Verification items for the finished model (mm, model axes). Face numbers are marked on the shaded views. A direction names the side the tool comes from. Give positions to 0.01 mm unless a question says otherwise; leave off trailing zeros. Order: outer loops, then holes, each group sorted by start corner. A loop starts at its lowest first (then second) coordinate and runs counter-clockwise, first axis right, second up.
from build123d import *

# Parameters (mm, degrees)
F1_DEPTH = 15
F2_R     = 2
F3_DEPTH = 5
F4_R     = 4
F5_R     = 2.1


with BuildPart() as f1:
    # F0 (on Top) → F1 (new body)
    with BuildSketch(Plane.XY):
        with BuildLine():
            ThreePointArc((3, -2.645751), (-3.741657, 1.414214), (4, 0))
            Line((4, 0), (4, -20.91608))
            Line((4, -20.91608), (6, -20.91608))
            Line((6, -20.91608), (6, 0))
            ThreePointArc((6, 0), (-4.582576, 3.872983), (1, -5.91608))
            Line((1, -5.91608), (1, -20.91608))
            Line((1, -20.91608), (3, -20.91608))
            Line((3, -20.91608), (3, -2.645751))
        make_face()
    extrude(amount=F1_DEPTH)

    # F2 (on face) → F3 (cut, through all)
    with BuildSketch(Plane(origin=(1, 0, 0), x_dir=(0, -1, 0), z_dir=(-1, 0, 0))):
        with Locations((13.41608, 7.5)):
            Circle(F2_R)
    extrude(amount=-F3_DEPTH, mode=Mode.SUBTRACT)

    # F4 (on face) → F6 section 0
    with BuildSketch(Plane(origin=(1, 0, 0), x_dir=(0, -1, 0), z_dir=(-1, 0, 0))):
        with Locations((13.41608, 7.5)):
            Circle(F4_R)
    # F5 (on face) → F6 section 1
    with BuildSketch(Plane.YZ.offset(3)):
        with Locations((-13.41608, 7.5)):
            Circle(F5_R)
    loft(mode=Mode.SUBTRACT)


solid = f1.part
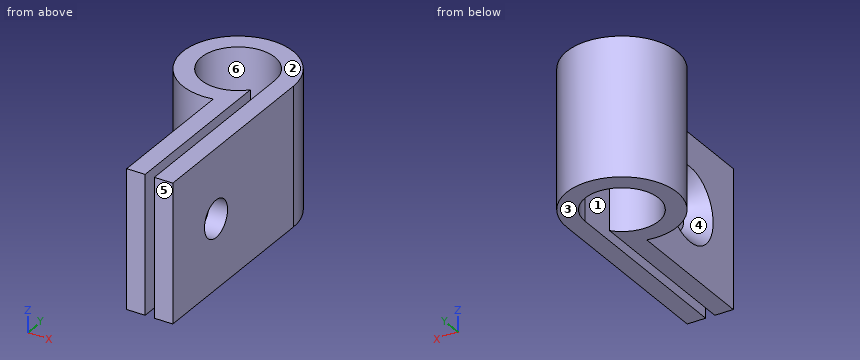
(1) Release check for a two-part mould opening along Y. For the marked faces 3, 4, 5 and 6 record: pulls with the +Y half, pulls with the -Y half, needs draft (parallel to the pull), parting line crosses it, or undercut.
Solved:
face 3: needs draft
face 4: undercut
face 5: pulls with the -Y half
face 6: undercut
(2) Scan lines: line 1 (X direction, y = -18.75, z = 3); line 2 (Y direction, x = 0, z = 9.75); line 3 (X direction, y = 0.5, z = 14). Record each from-to range of solid material in increasing order.
Solved:
line 1: x = 1 to 3, 4 to 6
line 2: y = -6 to -4, 4 to 6
line 3: x = -5.98 to -3.97, 3.97 to 5.98
(3) Go/stop test with flat-tipped pins: pin 1 (3.5 mm diameter, centred on y = -13.42, z = 7.5, fed in from +X); pin 2 (7.5 mm diameter, centred on y = -15.5, z = 7, fed in from -X). Record where each tip stops, or that it passes through.
Solved:
pin 1: passes through
pin 2: stops at x = 1
(4) Section check A-A, the plane y = -7.25. Enter the section's corners in (x, z).
Solved:
outline: (1, 0) - (3, 0) - (3, 15) - (1, 15) - close; (4, 0) - (6, 0) - (6, 15) - (4, 15) - close
(5) Section check C-C, the plane z = 14.25. Enter the section's corners in (x, y).
Solved:
outline: (1, -20.92) - (3, -20.92) - (3, -2.65) arc R4 cw (long way) to (4, 0) - (4, -20.92) - (6, -20.92) - (6, 0) arc R6 ccw (long way) to (1, -5.92) - close
(6) Section check B-B, the plane x = 0. Enter the section's corners in (y, z), then the cut area to 3 significant figures.
Solved:
outline: (-6, 0) - (-4, 0) - (-4, 15) - (-6, 15) - close; (4, 0) - (6, 0) - (6, 15) - (4, 15) - close
area: 60.0 mm2
(7) Set-up check for the marked faces 1 and 2: record each of +Z, -Z, +X, -X, +Y, -Y from which the full face is reachable in a straight line by a thin tool's end or side.
Solved:
face 1: +Z, -Z, -Y
face 2: +Z, +X, -X, +Y, -Y
(8) Section check D-D, the plane x = 4.75. Enter the section's corners in (y, z), then the cut area to 3 significant figures.
Solved:
outline: (-20.92, 0) - (3.67, 0) - (3.67, 15) - (-20.92, 15) - close; hole circle Ø4 at (-13.42, 7.5)
area: 356 mm2
